The model under review builds one solid part; all positions refer to its coordinate system, in mm. A direction names the side the tool comes from. Give positions to 0.01 mm unless a question says otherwise; leave off trailing zeros. Loops run counter-clockwise (first coordinate to the right, second up) from the corner with the lowest first, then second, coordinate; pieces in that order, holes last. Notation, with made-up numbers: (38.25, 44) -> (46.25, 44) arc R27 ccw to (46.25, 69) -> close; hole circle Ø1 at (59, -21.75). An arc over 180 degrees is marked (long way). Write each question's results on one line, items separated by ' | '. Start each with the question number.
Q1. We need section A-A (z = -3). Give the number of separate pieces and of enclosed holes in the cut face, plus the area to 3 significant figures.
Q2. We need section B-B (y = 19.25). Write out the cut boundary in (x, z).
Q3. Wall thickness on L1, parallel to Y at x = -0.5, z = 3.75; L2, parallel to Z at x = 2.5, y = 9; L3, parallel to Y at x = -3, z = 5.5: over which ranges is each line inside the solid? List them lowest first. Write a range as [from, to].
Q4. Machinability: for faces 1 (the face through (-0.623, 3.877, -4.747)), 2 (the face through (0, 0, 0)), which of the approach directions +Z, -Z, +X, -X, +Y, -Y give a long, thin tool a straight path to every point of the face, cutting with its end or side? Answer none if there is none.
Q5. We need section D-D (y = 15). Write out the cut boundary in (x, z), plus the area to 3 significant figures.
Q6. Insertion check: pin 1 Ø1 at (y, z) = (3.5, -1.5) entering from +X; pin 2 Ø1.5 at (y, z) = (2.5, 1) entering from -X; pin 3 Ø5 at (y, z) = (13.5, -1) entering from -X. Each pin has a flat end and moves straight along its axis. Give the tip position at first contact, or say it passes through.
from build123d import *


with BuildPart() as part:
    # Sketch1 → Revolve4 (revolve)
    with BuildSketch(Plane.XY):
        with BuildLine():
            Line((0, 0), (0, 20.718792279))
            ThreePointArc((0, 20.718792279), (3.264480019, 18.531398873), (2.482849316, 14.680350555))
            ThreePointArc((2.482849316, 14.680350555), (3.365856417, 13.797343455), (2.482849316, 12.914336354))
            add(Edge.make_bspline(
                [(2.482849316, 12.914336354), (2.583418025, 8.286863587), (4.787525553, 4.183965741)],
                knots=[0, 0, 0, 1, 1, 1], degree=2))
            Line((4.787525553, 4.183965741), (4.787525553, 3.578409965))
            ThreePointArc((4.787525553, 3.578409965), (5.560964983, 2.876116424), (5.611272713, 1.832615632))
            Line((5.611272713, 1.832615632), (6.35, 1.093888345))
            Line((6.35, 1.093888345), (6.35, 0))
            Line((6.35, 0), (0, 0))
        make_face()
    revolve(axis=Axis((0, 0, 0), (0, 1, 0)))


solid = part.part
Output:
1) separate pieces: 3 | enclosed holes: 0 | area: 75.1 mm2
2) outline: circle Ø5.73 at (0, 0)
3) L1: [0, 6.35] | L2: [-1.6, 1.6] | L3: [0, 1.18]
4) face 1: +Y | face 2: +Z, -Z, +X, -X, -Y
5) outline: circle Ø5.54 at (0, 0) | area: 24.1 mm2
6) pin 1: x = 5.31 | pin 2: x = -5.68 | pin 3: x = -3.37
